The listing builds one solid part. Answer for the finished solid, in the listing's coordinates (mm). Coordinates: 2 decimals unless noted, no trailing zeros. Order: outer loops, then holes, each group sorted by start corner. A loop starts at its lowest first (then second) coordinate and runs counter-clockwise, first axis right, second up. Notation, with made-up numbers: (-31, -24.75) - (15, -24.75) arc R10 cw to (15, -18.75) - close; hole circle Ø9 at (55.5, 50). An arc over 180 degrees is marked (long way). Use a Markdown table: item, result. Add a question column.
Item 1: The part is cut by section C-C, the plane z = 19.05. State how many separate pieces and enclosed holes the cut face has, then the cut area to 3 significant figures.
Item 2: The part is cut by section B-B, the plane x = -19.05. Give the vertices of the cut face in (y, z), then the cut area to 3 significant figures.
Item 3: The mould has two halves that part along X. Classify faces 1 (the cylindrical face through (-10.661, 4.542, 23.054)), 2 (the flat face through (5, 6.35, 0)), 3 (the cylindrical face through (-11.48, 3.22, 14.29)): released by +X, released by -X, zero draft, split by the parting line, or undercut.
Item 4: Find the intervals of material crossed by line 1 along X through (y, z) = (2.5, 0); line 2 along Z through (x, y) = (-12.5, 0.75), in increasing order.
Item 5: The part is cut by section A-A, the plane z = 0. Give the vertices of the cut face in (x, y), then the cut area to 3 significant figures.
Item 6: A flat-ended cylindrical pin translates along its axis: P1, Ø1.5, axis at y = 4, z = 17.5, coming from the -X side. Find the tip coordinate at first contact, or state that the pin passes through.
from build123d import *

# Parameters (mm, degrees)
SKETCH1_R              = 25.4
BOSS_EXTRUDE1_DEPTH    = 6.35
CUT_EXTRUDE2_REACH     = 8.35
SKETCH3_R              = 2.15265
SKETCH5_W              = 12.7
SKETCH5_H              = 6.35
CUT_EXTRUDE3_DEPTH     = 1.5875
F_4_40TAPPEDHOLE_REACH = 58.999
SKETCH6_R              = 1.1303
CUT_EXTRUDE5_REACH     = 8.35
SKETCH8_R              = 4


with BuildPart() as part:
    # Sketch1 → Boss-Extrude1 (new body)
    with BuildSketch(Plane(origin=(0, 0, 0), x_dir=(1, 0, 0), z_dir=(0, 1, 0))):
        Circle(SKETCH1_R)
    extrude(amount=BOSS_EXTRUDE1_DEPTH)

    # Sketch3 → Cut-Extrude2 (cut, up to next)
    with BuildSketch(Plane(origin=(0, 6.35, 0), x_dir=(1, 0, 0), z_dir=(0, 1, 0)), mode=Mode.PRIVATE) as cut_extrude2_sk1:
        with Locations((-13.470384182, 13.470384182)):
            Circle(SKETCH3_R)
    cut_extrude2_tool1 = extrude(cut_extrude2_sk1.sketch, amount=-CUT_EXTRUDE2_REACH, mode=Mode.PRIVATE) & part.part
    add(cut_extrude2_tool1.solids().sort_by_distance((-13.470384, 6.35, -13.470384))[0], mode=Mode.SUBTRACT)
    # Sketch3 → Cut-Extrude2 (cut, up to next)
    with BuildSketch(Plane(origin=(0, 6.35, 0), x_dir=(1, 0, 0), z_dir=(0, 1, 0)), mode=Mode.PRIVATE) as cut_extrude2_sk2:
        with Locations((0, 19.05)):
            Circle(SKETCH3_R)
    cut_extrude2_tool2 = extrude(cut_extrude2_sk2.sketch, amount=-CUT_EXTRUDE2_REACH, mode=Mode.PRIVATE) & part.part
    add(cut_extrude2_tool2.solids().sort_by_distance((0, 6.35, -19.05))[0], mode=Mode.SUBTRACT)
    # Sketch3 → Cut-Extrude2 (cut, up to next)
    with BuildSketch(Plane(origin=(0, 6.35, 0), x_dir=(1, 0, 0), z_dir=(0, 1, 0)), mode=Mode.PRIVATE) as cut_extrude2_sk3:
        with Locations((13.470384182, 13.470384182)):
            Circle(SKETCH3_R)
    cut_extrude2_tool3 = extrude(cut_extrude2_sk3.sketch, amount=-CUT_EXTRUDE2_REACH, mode=Mode.PRIVATE) & part.part
    add(cut_extrude2_tool3.solids().sort_by_distance((13.470384, 6.35, -13.470384))[0], mode=Mode.SUBTRACT)
    # Sketch3 → Cut-Extrude2 (cut, up to next)
    with BuildSketch(Plane(origin=(0, 6.35, 0), x_dir=(1, 0, 0), z_dir=(0, 1, 0)), mode=Mode.PRIVATE) as cut_extrude2_sk4:
        with Locations((19.05, 0)):
            Circle(SKETCH3_R)
    cut_extrude2_tool4 = extrude(cut_extrude2_sk4.sketch, amount=-CUT_EXTRUDE2_REACH, mode=Mode.PRIVATE) & part.part
    add(cut_extrude2_tool4.solids().sort_by_distance((19.05, 6.35, 0))[0], mode=Mode.SUBTRACT)
    # Sketch3 → Cut-Extrude2 (cut, up to next)
    with BuildSketch(Plane(origin=(0, 6.35, 0), x_dir=(1, 0, 0), z_dir=(0, 1, 0)), mode=Mode.PRIVATE) as cut_extrude2_sk5:
        with Locations((13.470384182, -13.470384182)):
            Circle(SKETCH3_R)
    cut_extrude2_tool5 = extrude(cut_extrude2_sk5.sketch, amount=-CUT_EXTRUDE2_REACH, mode=Mode.PRIVATE) & part.part
    add(cut_extrude2_tool5.solids().sort_by_distance((13.470384, 6.35, 13.470384))[0], mode=Mode.SUBTRACT)
    # Sketch3 → Cut-Extrude2 (cut, up to next)
    with BuildSketch(Plane(origin=(0, 6.35, 0), x_dir=(1, 0, 0), z_dir=(0, 1, 0)), mode=Mode.PRIVATE) as cut_extrude2_sk6:
        with Locations((0, -19.05)):
            Circle(SKETCH3_R)
    cut_extrude2_tool6 = extrude(cut_extrude2_sk6.sketch, amount=-CUT_EXTRUDE2_REACH, mode=Mode.PRIVATE) & part.part
    add(cut_extrude2_tool6.solids().sort_by_distance((0, 6.35, 19.05))[0], mode=Mode.SUBTRACT)
    # Sketch3 → Cut-Extrude2 (cut, up to next)
    with BuildSketch(Plane(origin=(0, 6.35, 0), x_dir=(1, 0, 0), z_dir=(0, 1, 0)), mode=Mode.PRIVATE) as cut_extrude2_sk7:
        with Locations((-13.470384182, -13.470384182)):
            Circle(SKETCH3_R)
    cut_extrude2_tool7 = extrude(cut_extrude2_sk7.sketch, amount=-CUT_EXTRUDE2_REACH, mode=Mode.PRIVATE) & part.part
    add(cut_extrude2_tool7.solids().sort_by_distance((-13.470384, 6.35, 13.470384))[0], mode=Mode.SUBTRACT)
    # Sketch3 → Cut-Extrude2 (cut, up to next)
    with BuildSketch(Plane(origin=(0, 6.35, 0), x_dir=(1, 0, 0), z_dir=(0, 1, 0)), mode=Mode.PRIVATE) as cut_extrude2_sk8:
        with Locations((-19.05, 0)):
            Circle(SKETCH3_R)
    cut_extrude2_tool8 = extrude(cut_extrude2_sk8.sketch, amount=-CUT_EXTRUDE2_REACH, mode=Mode.PRIVATE) & part.part
    add(cut_extrude2_tool8.solids().sort_by_distance((-19.05, 6.35, 0))[0], mode=Mode.SUBTRACT)

    # Sketch5 → Cut-Extrude3 (cut)
    with BuildSketch(Plane(origin=(9.720159182, 0, -23.466540126), x_dir=(-0.923879533, 0, -0.382683432), z_dir=(0.382683432, 0, -0.923879533))):
        with Locations((0, 3.175)):
            Rectangle(SKETCH5_W, SKETCH5_H)
    extrude(amount=-CUT_EXTRUDE3_DEPTH, mode=Mode.SUBTRACT)

    # Sketch6 → 4-40TappedHole (cut, up to next)
    with BuildSketch(Plane(origin=(9.112649233, 0, -21.999881368), x_dir=(-0.923879533, 0, -0.382683432), z_dir=(0.382683432, 0, -0.923879533)), mode=Mode.PRIVATE) as f_4_40tappedhole_sk1:
        with Locations((0, 3.175)):
            Circle(SKETCH6_R)
    f_4_40tappedhole_tool1 = extrude(f_4_40tappedhole_sk1.sketch, amount=-F_4_40TAPPEDHOLE_REACH, mode=Mode.PRIVATE) & part.part
    add(f_4_40tappedhole_tool1.solids().sort_by_distance((9.112649, 3.175, -21.999881))[0], mode=Mode.SUBTRACT)

    # Sketch8 → Cut-Extrude5 (cut, up to next)
    with BuildSketch(Plane(origin=(0, 6.35, 0), x_dir=(1, 0, 0), z_dir=(0, 1, 0)), mode=Mode.PRIVATE) as cut_extrude5_sk1:
        Circle(SKETCH8_R)
    cut_extrude5_tool1 = extrude(cut_extrude5_sk1.sketch, amount=-CUT_EXTRUDE5_REACH, mode=Mode.PRIVATE) & part.part
    add(cut_extrude5_tool1.solids().sort_by_distance((0, 6.35, 0))[0], mode=Mode.SUBTRACT)


solid = part.part
Solution:
| question | item | result |
|---|---|---|
| 1 | separate pieces | 2 |
| 1 | enclosed holes | 1 |
| 1 | area | 182 mm2 |
| 2 | outline | (0, -16.8) - (6.35, -16.8) - (6.35, -2.15) - (0, -2.15) - close; (0, 2.15) - (6.35, 2.15) - (6.35, 16.8) - (0, 16.8) - close |
| 2 | area | 186 mm2 |
| 3 | face 1 | split by the parting line |
| 3 | face 2 | zero draft |
| 3 | face 3 | undercut |
| 4 | line 1 | x = -25.4 to -21.2, -16.9 to -4, 4 to 16.9, 21.2 to 25.4 |
| 4 | line 2 | z = -22.11 to -15.39, -11.55 to 11.55, 15.39 to 22.11 |
| 5 | outline | (-25.4, 0) - (-21.2, 0) - (-21.2, 6.35) - (-25.4, 6.35) - close; (-16.9, 0) - (-4, 0) - (-4, 6.35) - (-16.9, 6.35) - close; (4, 0) - (16.9, 0) - (16.9, 6.35) - (4, 6.35) - close; (21.2, 0) - (25.4, 0) - (25.4, 6.35) - (21.2, 6.35) - close |
| 5 | area | 217 mm2 |
| 6 | P1 | stops at x = -19.09 |
